Could you check a few things on this model? Use its own coordinates, in mm. Face numbers are marked on the shaded views. A direction names the side the tool comes from. Round coordinates to 2 decimals unless told otherwise and drop trailing zeros. Write each loop counter-clockwise with the first axis right and the second up, starting at its lowest first coordinate (ties: lowest second). Pieces come first, ordered by that corner, then holes. Notation, with made-up numbers: (52.5, -9) - (104.5, -9) arc R9 ccw to (104.5, 5) - close; hole circle Ø2 at (-14, 46.5). An arc over 180 degrees is marked (long way). Put each result on its own line as item: value.
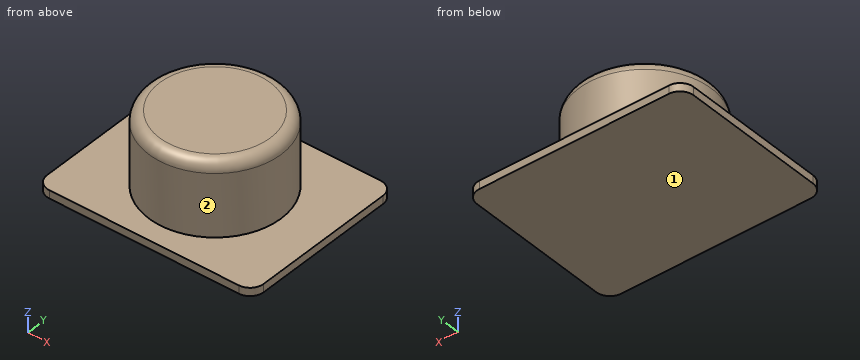
from build123d import *

# Parameters (mm, degrees)
SKETCH_W     = 80
SKETCH_H     = 63.5
PAD_DEPTH    = 3
SKETCH001_R  = 24.4
PAD001_DEPTH = 27
FILLET_R     = 4
FILLET001_R  = 5


with BuildPart() as part:
    # Sketch → Pad (new body)
    with BuildSketch(Plane.XY):
        Rectangle(SKETCH_W, SKETCH_H)
    extrude(amount=PAD_DEPTH)

    # Sketch001 (on Face6 of Pad) → Pad001 (join)
    with BuildSketch(Plane.XY.offset(3)):
        Circle(SKETCH001_R)
    extrude(amount=PAD001_DEPTH)

    # Fillet
    fillet_edges = [part.edges().sort_by_distance(p)[0] for p in [
        (-24.4, 0, 30),
    ]]
    fillet(fillet_edges, radius=FILLET_R)

    # Fillet001
    fillet001_edges = [part.edges().sort_by_distance(p)[0] for p in [
        (40, -31.75, 1.5),
        (40, 31.75, 1.5),
        (-40, 31.75, 1.5),
        (-40, -31.75, 1.5),
    ]]
    fillet(fillet001_edges, radius=FILLET001_R)


solid = part.part
(1) Please list where these lines run through material, in increasing order: probe 1 along Z at (x, y) = (26, -17); probe 2 along X at (y, z) = (1.5, 11); probe 3 along X at (y, z) = (-20, 15.5). Write a range as from..to.
Values found:
probe 1: z = 0..3
probe 2: x = -24.35..24.35
probe 3: x = -13.98..13.98
(2) I'm going to push flat-ended pins straight in: pin 1 (8 mm diameter, centred on x = -20.5, y = 23.5, fed in from -Z); pin 2 (4 mm diameter, centred on y = 2, z = 7, fed in from +X); pin 3 (3 mm diameter, centred on y = -20, z = 14, fed in from -X); pin 4 (6 mm diameter, centred on y = 14, z = 8.5, fed in from +X). Where does each tip first touch, or does it pass through?
Values found:
pin 1: stops at z = 0
pin 2: stops at x = 24.4
pin 3: stops at x = -15.91
pin 4: stops at x = 21.78
(3) Imagine slicing it at D-D, the plane x = 28.5. List the corners of the cut face in (y, z) for me, then the cut area to 4 significant figures.
Values found:
outline: (-31.75, 0) - (31.75, 0) - (31.75, 3) - (-31.75, 3) - close
area: 190.5 mm^2
(4) For the marked faces 1 and 2, which set-ups out of +Z, -Z, +X, -X, +Y, -Y let a thin tool reach every point of the face, with its end or its side?
Values found:
face 1: -Z, +X, -X, +Y, -Y
face 2: +Z
(5) Imagine slicing it at B-B, the plane x = 0. List the corners of the cut face in (y, z) for me, then the cut area to 3 significant figures.
Values found:
outline: (-31.75, 0) - (31.75, 0) - (31.75, 3) - (24.4, 3) - (24.4, 26) arc R4 ccw to (20.4, 30) - (-20.4, 30) arc R4 ccw to (-24.4, 26) - (-24.4, 3) - (-31.75, 3) - close
area: 1,500 mm^2
(6) Imagine slicing it at A-A, the plane y = 0. List the corners of the cut face in (x, z) for me.
Values found:
outline: (-40, 0) - (40, 0) - (40, 3) - (24.4, 3) - (24.4, 26) arc R4 ccw to (20.4, 30) - (-20.4, 30) arc R4 ccw to (-24.4, 26) - (-24.4, 3) - (-40, 3) - close
(7) Imagine slicing it at C-C, the plane z = 14.5. List the corners of the cut face in (x, y) for me.
Values found:
outline: circle Ø48.8 at (0, 0)
